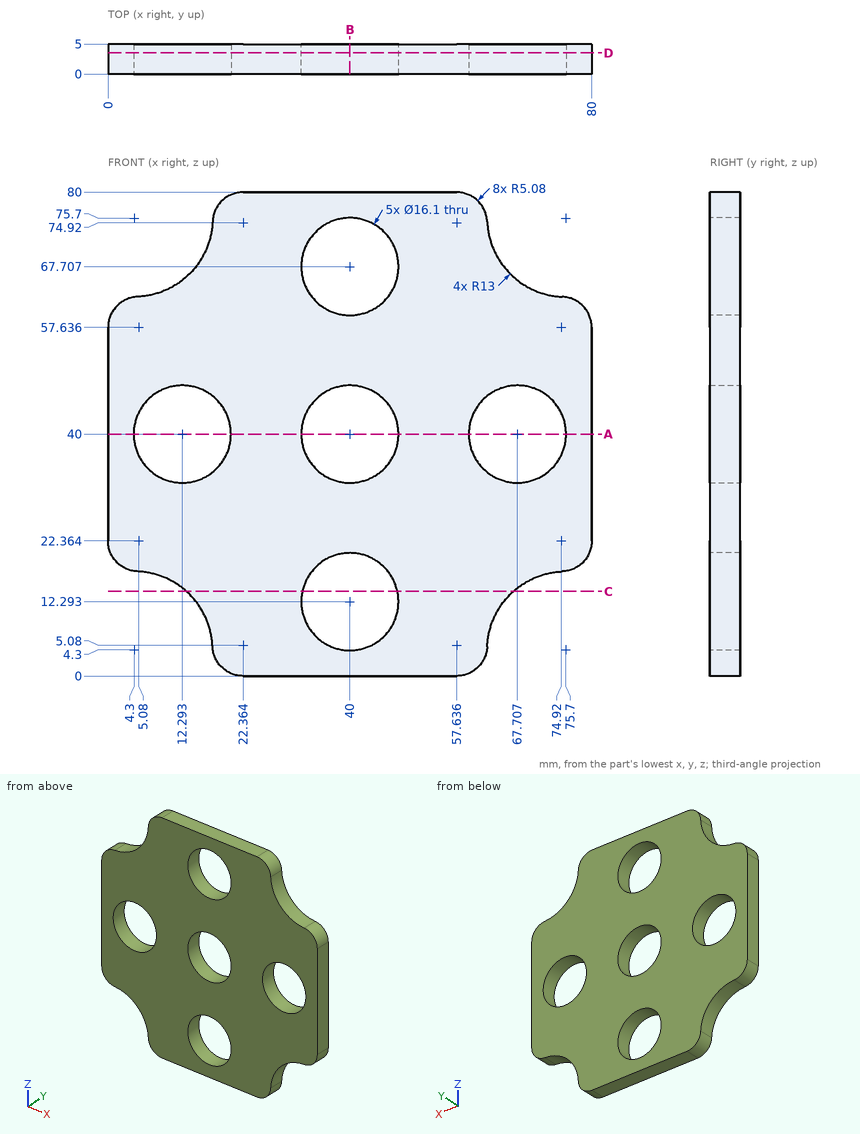
Check sheet for the drawn part. Datum: minimum x, y, z corner. Units: mm. Give positions to 0.01 mm unless a question says otherwise; leave off trailing zeros. Order: outer loops, then holes, each group sorted by start corner. A loop starts at its lowest first (then second) coordinate and runs counter-clockwise, first axis right, second up. Notation, with made-up numbers: (73.5, 27.25) - (92.5, 27.25) arc R13 cw to (92.5, 35.25) - close; hole circle Ø3 at (-27, 64). An arc over 180 degrees is marked (long way). Answer as a JSON object with one key per item and string values.
(1) Cross-section at A-A (z = 40). Record the cut outline in (x, y).
Report:
{"outline": "(0, 0) - (4.24, 0) - (4.24, 5) - (0, 5) - close; (20.34, 0) - (31.95, 0) - (31.95, 5) - (20.34, 5) - close; (48.05, 0) - (59.66, 0) - (59.66, 5) - (48.05, 5) - close; (75.76, 0) - (80, 0) - (80, 5) - (75.76, 5) - close"}
(2) Cross-section at B-B (x = 40). Record the cut outline in (y, z).
Report:
{"outline": "(0, 0) - (5, 0) - (5, 4.24) - (0, 4.24) - close; (0, 20.34) - (5, 20.34) - (5, 31.95) - (0, 31.95) - close; (0, 48.05) - (5, 48.05) - (5, 59.66) - (0, 59.66) - close; (0, 75.76) - (5, 75.76) - (5, 80) - (0, 80) - close"}
(3) Cross-section at D-D (y = 3.55). Record the cut outline in (x, z).
Report:
{"outline": "(0, 22.36) arc R5.08 ccw to (4.86, 17.29) arc R13 cw to (17.29, 4.86) arc R5.08 ccw to (22.36, 0) - (57.64, 0) arc R5.08 ccw to (62.71, 4.86) arc R13 cw to (75.14, 17.29) arc R5.08 ccw to (80, 22.36) - (80, 57.64) arc R5.08 ccw to (75.14, 62.71) arc R13 cw to (62.71, 75.14) arc R5.08 ccw to (57.64, 80) - (22.36, 80) arc R5.08 ccw to (17.29, 75.14) arc R13 cw to (4.86, 62.71) arc R5.08 ccw to (0, 57.64) - close; hole circle Ø16.1 at (12.29, 40); hole circle Ø16.1 at (40, 12.29); hole circle Ø16.1 at (40, 40); hole circle Ø16.1 at (40, 67.71); hole circle Ø16.1 at (67.71, 40)"}
(4) Cross-section at C-C (z = 14). Record the cut outline in (x, y).
Report:
{"outline": "(12.96, 0) - (32.13, 0) - (32.13, 5) - (12.96, 5) - close; (47.87, 0) - (67.04, 0) - (67.04, 5) - (47.87, 5) - close"}
(5) Material ranges on line 1 (Z direction, x = 40, y = 2.9); line 2 (Z direction, x = 12.5, y = 4.2) (1 decimal); line 3 (Z direction, x = 6, y = 2.15), recorded low to high.
Report:
{"line 1": "0 to 4.24, 20.34 to 31.95, 48.05 to 59.66, 75.76 to 80", "line 2": "14.4 to 32, 48 to 65.6", "line 3": "17.19 to 34.98, 45.02 to 62.81"}
(6) Depth check by flat-ended pin: pin 1 Ø3 at (y, z) = (1, 52.5) entering from -X; pin 2 Ø14.5 at (x, z) = (40, 67.71) entering from -Y. Enter the tip coordinate at first touch or a pass-through.
Report:
{"pin 1": "x = 0", "pin 2": "through"}
